```python
from build123d import *

# Parameters (mm, degrees)
SKETCH1_W               = 279.4
SKETCH1_H               = 76.2
BOSS_EXTRUDE1_DEPTH     = 3
SKETCH3_W               = 3
SKETCH3_H               = 15
CUT_EXTRUDE1_DEPTH      = 145.833352512
LPATTERN1_COUNT         = 3
LPATTERN1_PITCH         = 22.8
MIRROR1_COPY_1_SKETCH_W = 3
MIRROR1_COPY_1_SKETCH_H = 15
MIRROR1_COPY_1_DEPTH    = 145.833352512
MIRROR1_COPY_2_SKETCH_W = 3
MIRROR1_COPY_2_SKETCH_H = 15
MIRROR1_COPY_2_DEPTH    = 145.833352512
SKETCH6_W               = 3
SKETCH6_H               = 7.8
CUT_EXTRUDE2_DEPTH      = 145.833352512
LPATTERN2_COUNT         = 4
LPATTERN2_PITCH         = 22.8
SKETCH8_W               = 3
SKETCH8_H               = 7.8
BOSS_EXTRUDE2_DEPTH     = 3
LPATTERN4_COUNT         = 11
LPATTERN4_PITCH         = 22.8
SKETCH9_R               = 11
CUT_EXTRUDE3_DEPTH      = 146.651295909
F_6_CLEARANCE_HOLE1_D   = 3.7973
CUT_EXTRUDE4_REACH      = 147.651
SKETCH12_W              = 20.2
SKETCH12_H              = 6.7
F_6_CLEARANCE_HOLE2_D   = 3.7973


with BuildPart() as part:
    # Sketch1 → Boss-Extrude1 (new body)
    with BuildSketch(Plane(origin=(0, 0, 0), x_dir=(0, 0, -1), z_dir=(1, 0, 0))):
        Rectangle(SKETCH1_W, SKETCH1_H)
    extrude(amount=-BOSS_EXTRUDE1_DEPTH)

    # Sketch3 → Cut-Extrude1 (cut, through all)
    with BuildSketch(Plane.ZY.offset(3)):
        with Locations((133.2, 22.8)):
            Rectangle(SKETCH3_W, SKETCH3_H)
    cut_extrude1 = extrude(amount=-CUT_EXTRUDE1_DEPTH, mode=Mode.SUBTRACT)

    # LPattern1: Cut-Extrude1 ×3
    with Locations(*[(0, -i * LPATTERN1_PITCH, 0) for i in range(1, LPATTERN1_COUNT)]):
        add(cut_extrude1, mode=Mode.SUBTRACT)

    # Mirror1: Cut-Extrude1 across plane
    add(cut_extrude1.mirror(Plane.XY), mode=Mode.SUBTRACT)

    # Mirror1 copy 1 sketch → Mirror1 copy 1 (cut, through all)
    with BuildSketch(Plane(origin=(-3, -22.8, 0), x_dir=(0, 0, -1), z_dir=(-1, 0, 0))):
        with Locations((133.2, -22.8)):
            Rectangle(MIRROR1_COPY_1_SKETCH_W, MIRROR1_COPY_1_SKETCH_H)
    extrude(amount=-MIRROR1_COPY_1_DEPTH, mode=Mode.SUBTRACT)

    # Mirror1 copy 2 sketch → Mirror1 copy 2 (cut, through all)
    with BuildSketch(Plane(origin=(-3, -45.6, 0), x_dir=(0, 0, -1), z_dir=(-1, 0, 0))):
        with Locations((133.2, -22.8)):
            Rectangle(MIRROR1_COPY_2_SKETCH_W, MIRROR1_COPY_2_SKETCH_H)
    extrude(amount=-MIRROR1_COPY_2_DEPTH, mode=Mode.SUBTRACT)

    # Sketch6 → Cut-Extrude2 (cut, through all)
    with BuildSketch(Plane.ZY.offset(3)):
        with Locations((1.56, 34.2)):
            Rectangle(SKETCH6_W, SKETCH6_H)
    cut_extrude2 = extrude(amount=-CUT_EXTRUDE2_DEPTH, mode=Mode.SUBTRACT)

    # LPattern2: Cut-Extrude2 ×4
    with Locations(*[(0, -i * LPATTERN2_PITCH, 0) for i in range(1, LPATTERN2_COUNT)]):
        add(cut_extrude2, mode=Mode.SUBTRACT)

    # Sketch8 → Boss-Extrude2 (add)
    with BuildSketch(Plane(origin=(0, 38.1, 0), x_dir=(1, 0, 0), z_dir=(0, 1, 0))):
        with Locations((-1.5, 113)):
            Rectangle(SKETCH8_W, SKETCH8_H)
    boss_extrude2 = extrude(amount=BOSS_EXTRUDE2_DEPTH)

    # LPattern4: Boss-Extrude2 ×11, 1 skipped
    with Locations(*[(0, 0, i * LPATTERN4_PITCH) for i in range(1, LPATTERN4_COUNT) if i not in (5,)]):
        add(boss_extrude2)

    # Sketch9 → Cut-Extrude3 (cut, through all)
    with BuildSketch(Plane.ZY.offset(3)):
        with Locations((67.38, -18.8)):
            Circle(SKETCH9_R)
    extrude(amount=-CUT_EXTRUDE3_DEPTH, mode=Mode.SUBTRACT)

    # #6 Clearance Hole1 (through all)
    with Locations(Plane(origin=(0, 0, 0), x_dir=(0, 0, -1), z_dir=(1, 0, 0))):
        with Locations((28.9, -26.55), (28.9, -11.55), (-28.9, -11.55), (-28.9, -26.55)):
            Hole(F_6_CLEARANCE_HOLE1_D / 2)

    # Sketch12 → Cut-Extrude4 (cut, up to next)
    with BuildSketch(Plane.ZY.offset(3), mode=Mode.PRIVATE) as cut_extrude4_sk1:
        with Locations((-107.7, -15.8)):
            Rectangle(SKETCH12_W, SKETCH12_H)
    cut_extrude4_tool1 = extrude(cut_extrude4_sk1.sketch, amount=-CUT_EXTRUDE4_REACH, mode=Mode.PRIVATE) & part.part
    # Sketch12 → Cut-Extrude4 (cut, up to next)
    with BuildSketch(Plane.ZY.offset(3), mode=Mode.PRIVATE) as cut_extrude4_sk2:
        with Locations((107.7, -15.8)):
            Rectangle(SKETCH12_W, SKETCH12_H)
    cut_extrude4_tool2 = extrude(cut_extrude4_sk2.sketch, amount=-CUT_EXTRUDE4_REACH, mode=Mode.PRIVATE) & part.part
    add(cut_extrude4_tool1.solids().sort_by_distance((-3, -15.8, -107.7))[0], mode=Mode.SUBTRACT)
    add(cut_extrude4_tool2.solids().sort_by_distance((-3, -15.8, 107.7))[0], mode=Mode.SUBTRACT)

    # #6 Clearance Hole2 (through all)
    with Locations(Plane.ZY.offset(3)):
        with Locations((-107.7, -23.15), (-107.7, -8.45), (107.7, -23.15), (107.7, -8.45)):
            Hole(F_6_CLEARANCE_HOLE2_D / 2)


solid = part.part
```
The listing builds one solid part. Answer for the finished solid, in the listing's coordinates (mm). Give positions to 0.01 mm unless a question says otherwise; leave off trailing zeros. Order: outer loops, then holes, each group sorted by start corner. A loop starts at its lowest first (then second) coordinate and runs counter-clockwise, first axis right, second up.
Item 1: The part is cut by section A-A, the plane y = 26. Give the vertices of the cut face in (x, z), and give its area (3 significant figures).
From the geometry:
outline: (-3, -139.7) - (0, -139.7) - (0, -134.7) - (-3, -134.7) - close; (-3, -131.7) - (0, -131.7) - (0, 131.7) - (-3, 131.7) - close; (-3, 134.7) - (0, 134.7) - (0, 139.7) - (-3, 139.7) - close
area: 820 mm2
Item 2: Given pin 1 Ø17.5 at (y, z) = (-18.8, 67.38) entering from -X; pin 2 Ø1.5 at (x, z) = (-1, 1.5) entering from +Y; pin 3 Ø0.9 at (x, z) = (-1, 132.5) entering from +Y, each flat-ended and moving along its own axis, determine where each tip first touches the part or whether it passes through.
From the geometry:
pin 1: passes through
pin 2: stops at y = 30.3
pin 3: stops at y = 38.1
Item 3: For a pull along Z with two mould halves and no side action, classify faces 1 (the face through (0, 2, 2)), 2 (the face through (-1.52, -18.32, 56.39)) as pulls with the +Z half, pulls with the -Z half, needs draft (parallel to the pull), parting line crosses it, or undercut.
From the geometry:
face 1: needs draft
face 2: undercut
Item 4: Find the intervals of material crossed by probe 1 along Y at (x, z) = (-1.2, 3); probe 2 along Y at (x, z) = (-1.35, -107.7); probe 3 along Y at (x, z) = (-0.7, -28.9), in increasing order.
From the geometry:
probe 1: y = -30.3 to -15.3, -7.5 to 7.5, 15.3 to 30.3
probe 2: y = -38.1 to -25.05, -21.25 to -19.15, -12.45 to -10.35, -6.55 to 38.1
probe 3: y = -38.1 to -28.45, -24.65 to -13.45, -9.65 to 38.1
Item 5: The part is cut by section B-B, the plane x = -1.05. Count the separate pieces of the cut face and the enclosed holes in it, and give its area (3 significant figures).
From the geometry:
separate pieces: 1
enclosed holes: 19
area: 20,400 mm2
Item 6: The part is cut by section C-C, the plane z = 39. Give the vertices of the cut face in (x, y), and give its area (3 significant figures).
From the geometry:
outline: (-3, -38.1) - (0, -38.1) - (0, 38.1) - (-3, 38.1) - close
area: 229 mm2
